CAD build for the part. Positions are in the model's coordinates, mm. Give positions to 0.01 mm unless a question says otherwise; leave off trailing zeros. Loops run counter-clockwise (first coordinate to the right, second up) from the corner with the lowest first, then second, coordinate; pieces in that order, holes last.
Autodesk Inventor part; units mm, degrees
ref_plane "XZ Plane" through (0, 0, 0) normal (0, 1, 0) x (-1, 0, 0)
sketch "スケッチ1" plane through (0, 0, 0) normal (0, 1, 0) x (-1, 0, 0)
  circle A0 centre (0, 0) radius 15
  line L0 (31, 31) -> (-31, 31)
  line L1 (-31, 31) -> (-31, -31)
  line L2 (-31, -31) -> (31, -31)
  line L3 (31, -31) -> (31, 31)
  line L4 (31, 31) -> (-31, -31) construction
  line L5 (-31, 31) -> (31, -31) construction
  dimension "d0" = 30
  dimension "d1" = 62
  dimension "d2" = 62
extrude "押し出し1" add sketch "スケッチ1" along normal blind 16
properties part number "bearing2b"
1. Saw through at A-A, the plane z = 0. List the corners of the cut face in (x, y).
Responses:
outline: (-31, 0) - (-15, 0) - (-15, 16) - (-31, 16) - close; (15, 0) - (31, 0) - (31, 16) - (15, 16) - close
2. Pull direction Z, two halves, no side cores. Call faces 1 (the face through (0, 8, 31)), 2 (the face through (-31, 8, 0)), 3 (the face through (14.985, 7.888, -0.66)): released by +Z, released by -Z, zero draft, split by the parting line, or undercut.
Responses:
face 1: released by +Z
face 2: zero draft
face 3: undercut
3. Saw through at C-C, the plane y = 10. List the corners of the cut face in (x, z).
Responses:
outline: (-31, -31) - (31, -31) - (31, 31) - (-31, 31) - close; hole circle Ø30 at (0, 0)
4. Probe line 1 along Z through (x, y) = (0, 12.5); line 2 along Z through (x, y) = (6.5, 9.5); line 3 along X through (y, z) = (13, -2.5). List the from-to ranges inside material, lowest first.
Responses:
line 1: z = -31 to -15, 15 to 31
line 2: z = -31 to -13.52, 13.52 to 31
line 3: x = -31 to -14.79, 14.79 to 31
5. Saw through at B-B, the plane x = 0. List the corners of the cut face in (y, z).
Responses:
outline: (0, -31) - (16, -31) - (16, -15) - (0, -15) - close; (0, 15) - (16, 15) - (16, 31) - (0, 31) - close
6. Drop flat-ended pins along their axis: pin 1 (12 mm diameter, centred on x = 5.5, z = -4.5, fed in from +Y); pin 2 (12 mm diameter, centred on x = -8, z = -4.5, fed in from +Y). Give the stop position or say it passes through.
Responses:
pin 1: passes through
pin 2: stops at y = 16
